from build123d import *

# Parameters (mm, degrees)
SKETCH1_R               = 4.7625
BOSS_EXTRUDE1_DEPTH     = 5.08
SKETCH4_W               = 19.05
SKETCH4_H               = 5.08
BOSS_EXTRUDE2_DEPTH     = 5.08
SKETCH5_R               = 1.651
SKETCH5_R_2             = 1.660728382
CUT_EXTRUDE1_DEPTH      = 1.0000001
CUT_EXTRUDE1_DEPTH_BACK = 6.0800001
SKETCH6_R               = 4.7625
BOSS_EXTRUDE3_DEPTH     = 5.08


with BuildPart() as part:
    # Sketch1 → Boss-Extrude1 (new body)
    with BuildSketch(Plane(origin=(0, 0, 0), x_dir=(1, 0, 0), z_dir=(0, 1, 0))):
        with BuildLine():
            Line((-9.525, 53.975), (9.525, 53.975))
            Line((9.525, 53.975), (9.525, 51.435))
            add(Edge.make_bspline(
                [(9.525, 51.435), (9.525, 51.21454564), (27.819109584, -48.895), (60.325, -48.895)],
                knots=[0, 0, 0, 0, 1, 1, 1, 1], degree=3))
            Line((60.325, -48.895), (-9.525, -48.895))
            Line((-9.525, -48.895), (-9.525, 53.975))
        make_face()
        with Locations((0, 45.9867)):
            Circle(SKETCH1_R, mode=Mode.SUBTRACT)
    extrude(amount=BOSS_EXTRUDE1_DEPTH)

    # Sketch4 → Boss-Extrude2 (add)
    with BuildSketch(Plane(origin=(0, 5.08, 0), x_dir=(1, 0, 0), z_dir=(0, 1, 0))):
        with Locations((50.8, -51.435)):
            Rectangle(SKETCH4_W, SKETCH4_H)
    extrude(amount=-BOSS_EXTRUDE2_DEPTH)

    # Sketch5 → Cut-Extrude1 (cut, two sides)
    with BuildSketch(Plane.XZ) as cut_extrude1_sk:
        with Locations((34.925, 40.005)):
            Circle(SKETCH5_R)
        with Locations((-3.175, 4.445)):
            Circle(SKETCH5_R_2)
    extrude(amount=CUT_EXTRUDE1_DEPTH, mode=Mode.SUBTRACT)
    extrude(cut_extrude1_sk.sketch, amount=-CUT_EXTRUDE1_DEPTH_BACK, mode=Mode.SUBTRACT)

    # Sketch6 → Boss-Extrude3 (add)
    with BuildSketch(Plane.XZ):
        with BuildLine():
            Line((-14.535912, -0.037592), (-9.525, -0.037592))
            Line((-9.525, -0.037592), (-9.525, -1.398441508))
            ThreePointArc((-9.525, -1.398441508), (-4.629912, -9.943592), (-9.525, -18.488742492))
            Line((-9.525, -18.488742492), (-9.525, -19.849592))
            Line((-9.525, -19.849592), (-14.535912, -19.849592))
            ThreePointArc((-14.535912, -19.849592), (-24.441912, -9.943592), (-14.535912, -0.037592))
        make_face()
        with Locations((-14.535912, -9.943592)):
            Circle(SKETCH6_R, mode=Mode.SUBTRACT)
    extrude(amount=-BOSS_EXTRUDE3_DEPTH)


solid = part.part
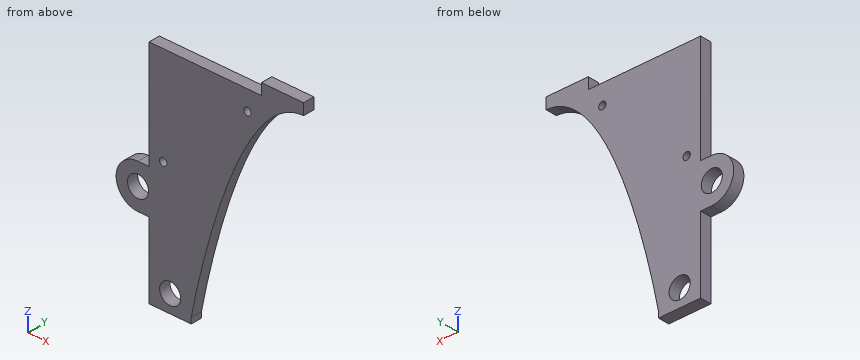
Model file for the job. Use its own axes, mm. Give positions to 0.01 mm unless a question says otherwise; leave off trailing zeros. Loops run counter-clockwise (first coordinate to the right, second up) from the corner with the lowest first, then second, coordinate; pieces in that order, holes last.
1) Saw through at A-A (x = 0). Write the cut outline in (y, z) (3 decimals).
2) Saw through at B-B (y = 1.05). Count the separate pieces of the cut face and the enclosed holes in it, plus the area to 3 significant figures.
3) Wall check: line 1 (Z direction, x = -18, y = 4.1); line 2 (Z direction, x = -8.5, y = 1.9) (3 decimals); line 3 (Z direction, x = 34, y = 2.2) (3 decimals). Give the ranges that are in metal, low to high.
4) Flat gauge pins, fed straight in: pin 1 Ø1 at (y, z) = (1.5, -38) entering from -X (3 decimals); pin 2 Ø1.3 at (y, z) = (2, -53.5) entering from +X (3 decimals); pin 3 Ø10 at (x, z) = (36.5, 28.5) entering from -Y; pin 4 Ø2.5 at (x, y) = (9, 2) entering from +Z (3 decimals). Where does each tip first touch, or does it go through?
Answer block:
1. outline: (0, -53.975) - (5.08, -53.975) - (5.08, -50.749) - (0, -50.749) - close; (0, -41.224) - (5.08, -41.224) - (5.08, 48.895) - (0, 48.895) - close
2. separate pieces: 1
2. enclosed holes: 4
2. area: 3,720 mm2
3. line 1: z = -19.22 to -13.21, -6.68 to -0.66
3. line 2: z = -53.975 to 48.895
3. line 3: z = 25.411 to 38.637, 41.373 to 48.895
4. pin 1: stops at x = -9.525
4. pin 2: stops at x = 9.525
4. pin 3: stops at y = 0
4. pin 4: stops at z = 48.895
